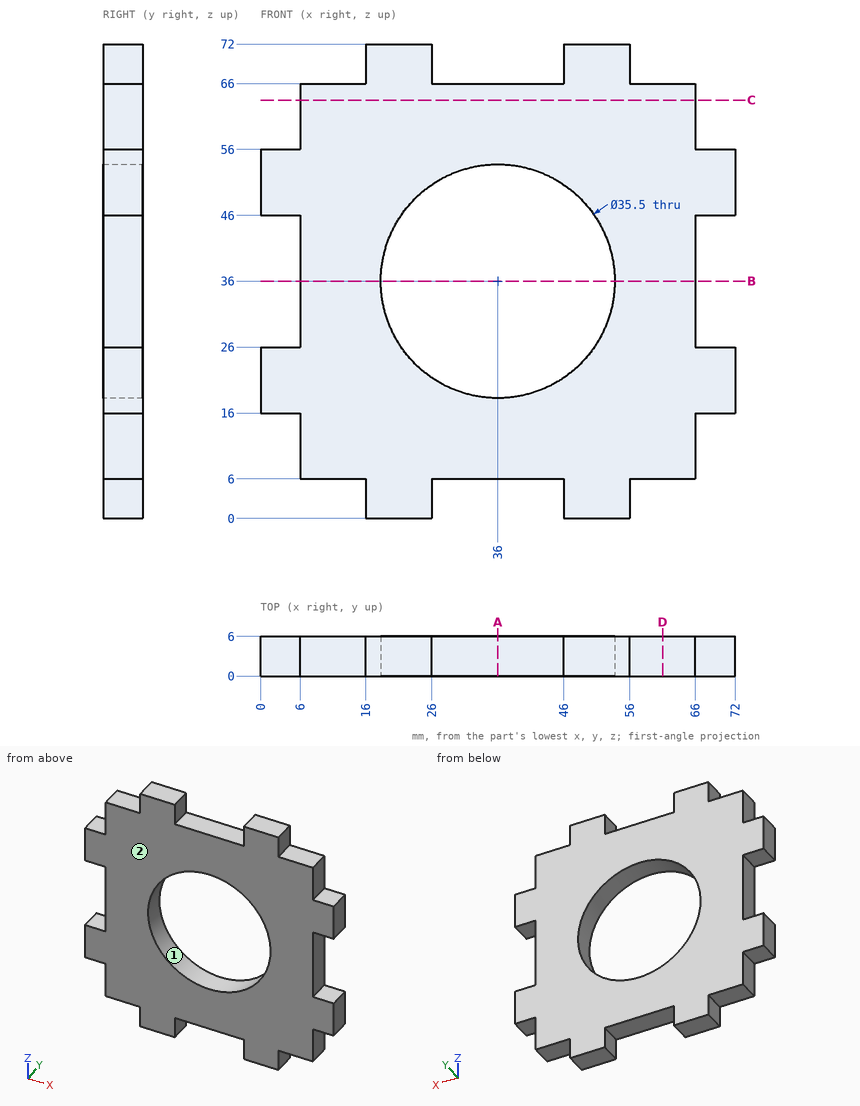
Study the drawing (mm; zero at the part's minimum x, y, z) and answer. Coordinates: 2 decimals unless noted, no trailing zeros. Order: outer loops, then holes, each group sorted by start corner. A loop starts at its lowest first (then second) coordinate and runs counter-clockwise, first axis right, second up. Notation, with made-up numbers: (63.25, 13.25) -> (95.25, 13.25) arc R29 cw to (95.25, 41.25) -> close; hole circle Ø8 at (51.5, 13). An arc over 180 degrees is marked (long way). Answer in a Markdown table with one row per item. Add a question column.
Item 1: Find the intervals of material crossed by L1, parallel to X at y = 4.6, z = 36; L2, parallel to Z at x = 33.5, y = 0.9; L3, parallel to Z at x = 49.5, y = 1.7, in increasing order. Write a range as from..to.
Item 2: Find section B-B (z = 36). Write down the section's boundary in (x, y).
Item 3: Each of these flat-tipped pins is pushed along its axis until it touches: P1, Ø1.8, axis at x = 67.5, y = 3, coming from the -Z side; P2, Ø1.8, axis at y = 1.5, z = 3.5, coming from the -X side; P3, Ø1.8, axis at x = 63, y = 2.5, coming from the +Z side. Where does it stop, or does it pass through?
Item 4: Find section D-D (x = 61). Write down the section's boundary in (y, z), then the cut area to 3 significant figures.
Item 5: Determine the mould class of the marked faces 1 and 2 for opening direction X: +X half, -X half, draft (parallel to the pull), parting line (faces both ways), or undercut.
Item 6: Find section A-A (x = 36). Write down the section's boundary in (y, z).
Item 7: Find section C-C (z = 63.5). Write down the section's boundary in (x, y).
Result set:
| question | item | result |
|---|---|---|
| 1 | L1 | x = 6..18.25, 53.75..66 |
| 1 | L2 | z = 6..18.43, 53.57..66 |
| 1 | L3 | z = 0..24.48, 47.52..72 |
| 2 | outline | (6, 0) -> (18.25, 0) -> (18.25, 6) -> (6, 6) -> close; (53.75, 0) -> (66, 0) -> (66, 6) -> (53.75, 6) -> close |
| 3 | P1 | stops at z = 16 |
| 3 | P2 | stops at x = 16 |
| 3 | P3 | stops at z = 66 |
| 4 | outline | (0, 6) -> (6, 6) -> (6, 66) -> (0, 66) -> close |
| 4 | area | 360 mm² |
| 5 | face 1 | undercut |
| 5 | face 2 | draft |
| 6 | outline | (0, 6) -> (6, 6) -> (6, 18.25) -> (0, 18.25) -> close; (0, 53.75) -> (6, 53.75) -> (6, 66) -> (0, 66) -> close |
| 7 | outline | (6, 0) -> (66, 0) -> (66, 6) -> (6, 6) -> close |
